```python
from build123d import *

# Parameters (mm, degrees)
SKETCH1_W           = 194.591670797
SKETCH1_H           = 20
SKETCH1_R           = 1.5
SKETCH1_W_2         = 182.591670797
SKETCH1_H_2         = 12
BOSS_EXTRUDE1_DEPTH = 3
CUT_EXTRUDE1_DEPTH  = 196.639766774
FILLET1_R           = 5


with BuildPart() as part:
    # Sketch1 → Boss-Extrude1 (new body)
    with BuildSketch(Plane(origin=(0, 0, 0), x_dir=(1, 0, 0), z_dir=(0, 1, 0))):
        with Locations((97.295835399, 10)):
            Rectangle(SKETCH1_W, SKETCH1_H)
        with Locations(Location((3, 17, 0), (0, 0, 270))):
            Circle(SKETCH1_R, mode=Mode.SUBTRACT)
        with Locations(Location((3, 3, 0), (0, 0, 90))):
            Circle(SKETCH1_R, mode=Mode.SUBTRACT)
        with Locations(Location((191.591670797, 3, 0), (0, 0, 270))):
            Circle(SKETCH1_R, mode=Mode.SUBTRACT)
        with Locations(Location((191.591670797, 17, 0), (0, 0, 90))):
            Circle(SKETCH1_R, mode=Mode.SUBTRACT)
        with Locations((97.295835399, 10)):
            Rectangle(SKETCH1_W_2, SKETCH1_H_2, mode=Mode.SUBTRACT)
    extrude(amount=BOSS_EXTRUDE1_DEPTH)

    # Sketch2 → Cut-Extrude1 (cut, through all)
    with BuildSketch(Plane(origin=(0, 3, 0), x_dir=(1, 0, 0), z_dir=(0, 1, 0))):
        Polygon((175.591670797, 17), (175.591670797, 16), (188.591670797, 16), (188.591670797, 4), (175.591670797, 4), (175.591670797, 3), (189.591670797, 3), (189.591670797, 17), align=None)
    extrude(amount=-CUT_EXTRUDE1_DEPTH, mode=Mode.SUBTRACT)

    # Fillet1
    # the kernel refuses this fillet: 5 mm, written as the material it adds along each edge
    with BuildSketch(Plane(origin=(189.591670797, 3, -17), x_dir=(0, 0, 1), z_dir=(0, -1, 0)), Plane(origin=(189.591670797, 3, -3), x_dir=(-1, 0, 0), z_dir=(0, -1, 0)), Plane(origin=(6, 0, -16), x_dir=(0, 0, 1), z_dir=(0, 1, 0))) as fillet1_piece_1:
        with BuildLine():
            CenterArc((FILLET1_R, FILLET1_R), FILLET1_R, 180, 90)
            Line((0, FILLET1_R), (-FILLET1_R * 0.02, FILLET1_R))
            Line((-FILLET1_R * 0.02, FILLET1_R), (-FILLET1_R * 0.02, -FILLET1_R * 0.02))
            Line((-FILLET1_R * 0.02, -FILLET1_R * 0.02), (FILLET1_R, -FILLET1_R * 0.02))
            Line((FILLET1_R, -FILLET1_R * 0.02), (FILLET1_R, 0))
        make_face()
    extrude(amount=3)
    with BuildSketch(Plane(origin=(175.591670797, 3, -17), x_dir=(1, 0, 0), z_dir=(0, -1, 0))) as fillet1_piece_2:
        with BuildLine():
            CenterArc((3, 5), FILLET1_R, 233.130102354, 36.869897646)
            Line((0, 1), (-0.06, 0.92))
            ThreePointArc((-0.06, 0.92), (-0.1, 0.5), (-0.1, 0))
            Line((-0.1, 0), (0, -0.1))
            Line((0, -0.1), (3, -0.1))
            Line((3, -0.1), (3, 0))
        make_face()
    extrude(amount=3)
    with BuildSketch(Plane(origin=(175.591670797, 3, -3), x_dir=(0, 0, -1), z_dir=(0, -1, 0))) as fillet1_piece_3:
        with BuildLine():
            CenterArc((5, 3), FILLET1_R, 180, 36.869897646)
            Line((0, 3), (-0.1, 3))
            Line((-0.1, 3), (-0.1, 0))
            Line((-0.1, 0), (0, -0.1))
            ThreePointArc((0, -0.1), (0.5, -0.1), (0.92, -0.06))
            Line((0.92, -0.06), (1, 0))
        make_face()
    extrude(amount=3)
    with BuildSketch(Plane(origin=(6, 0, -4), x_dir=(0, 0, -1), z_dir=(0, 1, 0))) as fillet1_piece_4:
        with BuildLine():
            CenterArc((FILLET1_R, -FILLET1_R), FILLET1_R, 90, 90)
            Line((0, -FILLET1_R), (-FILLET1_R * 0.02, -FILLET1_R))
            Line((-FILLET1_R * 0.02, -FILLET1_R), (-FILLET1_R * 0.02, FILLET1_R * 0.02))
            Line((-FILLET1_R * 0.02, FILLET1_R * 0.02), (FILLET1_R, FILLET1_R * 0.02))
            Line((FILLET1_R, FILLET1_R * 0.02), (FILLET1_R, 0))
        make_face()
    extrude(amount=3)


solid = part.part
```
Geometry: final body of the model. Coordinates: model frame, mm. A direction names the side the tool comes from. Round coordinates to 2 decimals unless told otherwise and drop trailing zeros. Order: outer loops, then holes, each group sorted by start corner. A loop starts at its lowest first (then second) coordinate and runs counter-clockwise, first axis right, second up. Notation, with made-up numbers: (35.5, 8.25) - (94.5, 8.25) arc R22 ccw to (94.5, 46.25) - close; hole circle Ø5 at (24.5, 65.5). An arc over 180 degrees is marked (long way). Write item = value, one per line. Start each with the question number.
Q1. Access query for faces 5 (the flat face through (189.592, 2, -10)), 6 (the flat face through (96, 0, -17)). Directions: +Z, -Z, +X, -X, +Y, -Y. A direction counts if a zero-diameter tool reaches every point of the face in a straight line with its end or side. Return the directions, or none.
Q2. Ray query, line 1 (Z direction, x = 128.5, y = 2.2); line 2 (X direction, y = 0.55, z = -8.5); line 3 (Z direction, x = 178, y = 0.75). Return the intervals inside material, ascending. Write a range as from..to.
Q3. Pull-direction query (Z, two-part tool) for faces 1 (the flat face through (194.592, 1, -10)), 2 (the flat face through (96, 1, -20)), 3 (the cylindrical face through (177.03, 1.52, -3.25)), 4 (the flat face through (96, 1, 0)); classes: +Z half, -Z half, draft (parallel to the pull), parting line (faces both ways), or undercut.
Q4. Cut plane A-A on x = 132.5. Return the cut outline in (y, z), and give its area (3 significant figures).
Q5. Pin query (flat end, axial travel): pin 1 (8 mm diameter, centred on x = 102.5, z = -15.5, fed in from +Y); pin 2 (2.5 mm diameter, centred on x = 191.59, z = -17, fed in from +Y). Return the tip coordinate at first contact, or that it passes through.
Q6. Cut plane B-B on y = 0.8. Return the cut outline in (x, z).
Outcome:
q1.face_5 = +Y, -Y
q1.face_6 = +Z, -Z, +X, -X, -Y
q2.line_1 = -20..-16, -4..0
q2.line_2 = 0..6.03, 189.59..194.59
q2.line_3 = -20..-16.96, -3.04..0
q3.face_1 = draft
q3.face_2 = -Z half
q3.face_3 = undercut
q3.face_4 = +Z half
q4.outline = (0, -20) - (3, -20) - (3, -16) - (0, -16) - close; (0, -4) - (3, -4) - (3, 0) - (0, 0) - close
q4.area = 24.0 mm^2
q5.pin_1 = 3
q5.pin_2 = through
q6.outline = (0, -20) - (194.59, -20) - (194.59, 0) - (0, 0) - close; hole circle Ø3 at (3, -17); hole circle Ø3 at (3, -3); hole (6, -11) arc R5 ccw to (11, -16) - (175.59, -16) arc R5 ccw to (178.59, -17) - (184.59, -17) arc R5 ccw to (189.59, -12) - (189.59, -8) arc R5 ccw to (184.59, -3) - (178.59, -3) arc R5 ccw to (175.59, -4) - (11, -4) arc R5 ccw to (6, -9) - close; hole circle Ø3 at (191.59, -17); hole circle Ø3 at (191.59, -3)
